```python
from build123d import *

# Parameters (mm, degrees)
ROTATION2_ANGLE                      = 36
SKIZZE3_R                            = 1
SCHNITT_LINEAR_AUSTRAGEN2_DEPTH      = 3.4
SCHNITT_LINEAR_AUSTRAGEN2_DEPTH_BACK = 21.661746393


with BuildPart() as part:
    # Skizze2 → Rotation2 (revolve, symmetric)
    with BuildSketch(Plane.XY) as rotation2_sk:
        with BuildLine():
            Line((-55.5, 3.250518846), (-58.158861149, 1.388764226))
            ThreePointArc((-58.158861149, 1.388764226), (-58.409608667, 1.102841481), (-58.5, 0.73344259))
            Line((-58.5, 0.73344259), (-58.5, -0.73344259))
            ThreePointArc((-58.5, -0.73344259), (-58.409608667, -1.102841481), (-58.158861149, -1.388764226))
            Line((-58.158861149, -1.388764226), (-55.5, -3.250518846))
            Line((-55.5, -3.250518846), (-55.5, -6.65))
            Line((-55.5, -6.65), (-61, -6.65))
            Line((-61, -6.65), (-61, 6.65))
            Line((-61, 6.65), (-55.5, 6.65))
            Line((-55.5, 6.65), (-55.5, 3.250518846))
        make_face()
    revolve(axis=Axis((0, 6.707883832, 0), (0, -1, 0)), revolution_arc=ROTATION2_ANGLE / 2)
    revolve(rotation2_sk.sketch, axis=Axis((0, 6.707883832, 0), (0, 1, 0)), revolution_arc=ROTATION2_ANGLE / 2)

    # Skizze3 → Schnitt-Linear austragen2 (cut, two sides)
    with BuildSketch(Plane(origin=(-58.014447494, 0, 0), x_dir=(0, 0, -1), z_dir=(1, 0, 0))) as schnitt_linear_austragen2_sk:
        with Locations(Location((0, 3.65, 0), (0, 0, 336.454253056))):
            Circle(SKIZZE3_R)
        with Locations(Location((0, -3.65, 0), (0, 0, 23.545976094))):
            Circle(SKIZZE3_R)
    extrude(amount=SCHNITT_LINEAR_AUSTRAGEN2_DEPTH, mode=Mode.SUBTRACT)
    extrude(schnitt_linear_austragen2_sk.sketch, amount=-SCHNITT_LINEAR_AUSTRAGEN2_DEPTH_BACK, mode=Mode.SUBTRACT)


solid = part.part
```
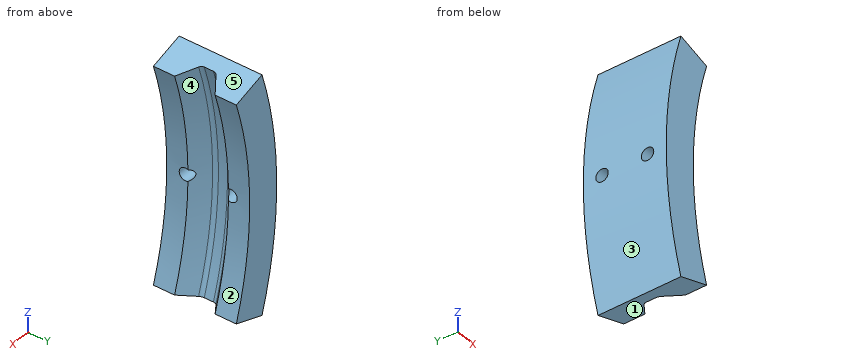
Verification items for the finished model (mm, model axes). Face numbers are marked on the shaded views. A direction names the side the tool comes from. Round coordinates to 2 decimals unless told otherwise and drop trailing zeros. Write each loop counter-clockwise with the first axis right and the second up, starting at its lowest first coordinate (ties: lowest second). Pieces come first, ordered by that corner, then holes.
1. Gauge pin test, flat ends, axial feed: P1, Ø1.5, axis at y = 1.5, z = 14.5, coming from the -X side; P2, Ø4, axis at x = -56, y = 2.5, coming from the -Z side; P3, Ø6, axis at y = 1, z = -3.5, coming from the -X side. Record the tip position at first contact, or that the pin passes through.
2. Draft check along Z on the marked faces 1, 2 and 3. Enter one of: +Z half, -Z half, draft (parallel to the pull), parting line (faces both ways), or undercut.
3. Section check B-B on z = 0. Enter the section's corners in (x, y), plus the area to 3 significant figures.
4. Access from +Z, -Z, +X, -X, +Y, -Y to the whole of each face (thin tool, end or side, straight path). Record for the marked faces 4 and 5.
5. Scan lines: L1, parallel to Y at x = -59.55, z = 0; L2, parallel to Y at x = -58.1, z = 0; L3, parallel to Z at x = -56.6, y = 3.65. Record each from-to range of solid material in increasing order.
6. Section check A-A on y = 3.65. Enter the section's corners in (x, z), plus the area to 3 significant figures.
7. Section check C-C on x = -59.5. Enter the section's corners in (y, z).
8. Section check D-D on y = -5.25. Enter the section's corners in (x, z).
Answer:
1. P1: stops at x = -59.43
1. P2: stops at z = -18.85
1. P3: stops at x = -61
2. face 1: -Z half
2. face 2: undercut
2. face 3: parting line
3. outline: (-61, -6.65) - (-55.5, -6.65) - (-55.5, -4.65) - (-61, -4.65) - close; (-61, -2.65) - (-56.36, -2.65) - (-58.16, -1.39) arc R0.8 cw to (-58.5, -0.73) - (-58.5, 0.73) arc R0.8 cw to (-58.16, 1.39) - (-56.36, 2.65) - (-61, 2.65) - close; (-61, 4.65) - (-55.5, 4.65) - (-55.5, 6.65) - (-61, 6.65) - close
3. area: 38.5 mm2
4. face 4: +X
4. face 5: +Z, +X, +Y, -Y
5. L1: y = -6.65 to -4.65, -2.65 to 2.65, 4.65 to 6.65
5. L2: y = -6.65 to -4.65, -2.65 to -1.43, 1.43 to 2.65, 4.65 to 6.65
5. L3: z = -18.39 to -1, 1 to 18.39
6. outline: (-60.99, -1) arc R61 ccw to (-58.01, -18.85) - (-52.78, -17.15) arc R55.5 cw to (-55.49, -1) - close; (-60.99, 1) - (-55.49, 1) arc R55.5 cw to (-52.78, 17.15) - (-58.01, 18.85) arc R61 ccw to start
6. area: 190 mm2
7. outline: (-6.65, -13.44) - (6.65, -13.44) - (6.65, 13.44) - (-6.65, 13.44) - close; hole circle Ø2 at (-3.65, 0); hole circle Ø2 at (3.65, 0)
8. outline: (-58.01, -18.85) - (-52.78, -17.15) arc R55.5 cw to (-52.78, 17.15) - (-58.01, 18.85) arc R61 ccw to start
